```python
from build123d import *

# Parameters (mm, degrees)
SKETCH1_R           = 25
BOSS_EXTRUDE1_DEPTH = 60
CUT_EXTRUDE1_DEPTH  = 60
SKETCH2_3_R         = 25
BOSS_EXTRUDE2_DEPTH = 120.5
FILLET1_R           = 12


with BuildPart() as part:
    # Sketch1 → Boss-Extrude1 (new body)
    with BuildSketch(Plane.XY):
        with BuildLine():
            Line((60, 30), (180, 30))
            Line((180, 30), (180, -30))
            Line((180, -30), (60, -30))
            ThreePointArc((60, -30), (44.188611699, -32.565835097), (30, -40))
            ThreePointArc((30, -40), (-50, 0), (30, 40))
            ThreePointArc((30, 40), (44.188611699, 32.565835097), (60, 30))
        make_face()
        Circle(SKETCH1_R, mode=Mode.SUBTRACT)
    extrude(amount=BOSS_EXTRUDE1_DEPTH)

    # Sketch2 → Cut-Extrude1 (cut)
    with BuildSketch(Plane(origin=(180, 0, 0), x_dir=(0, 0, -1), z_dir=(1, 0, 0))):
        Polygon((-60, 11.94), (-41.94, 30), (-60, 30), align=None)
        Polygon((0, -30), (0, -11.94), (-18.06, -30), align=None)
        Polygon((0, 30), (-18.06, 30), (0, 11.94), align=None)
        Polygon((-41.94, -30), (-60, -11.94), (-60, -30), align=None)
    extrude(amount=-CUT_EXTRUDE1_DEPTH, mode=Mode.SUBTRACT)

    # Sketch2_3 → Boss-Extrude2 (add)
    with BuildSketch(Plane(origin=(180, 0, 0), x_dir=(0, 0, -1), z_dir=(1, 0, 0))):
        with Locations((-30, 0)):
            Circle(SKETCH2_3_R)
    extrude(amount=BOSS_EXTRUDE2_DEPTH)

    # Fillet1
    fillet1_edges = [part.edges().sort_by_distance(p)[0] for p in [
        (120, -20.97, 50.97),
        (120, 20.97, 9.03),
        (120, -20.97, 9.03),
        (120, 20.97, 50.97),
    ]]
    fillet(fillet1_edges, radius=FILLET1_R)


solid = part.part
```
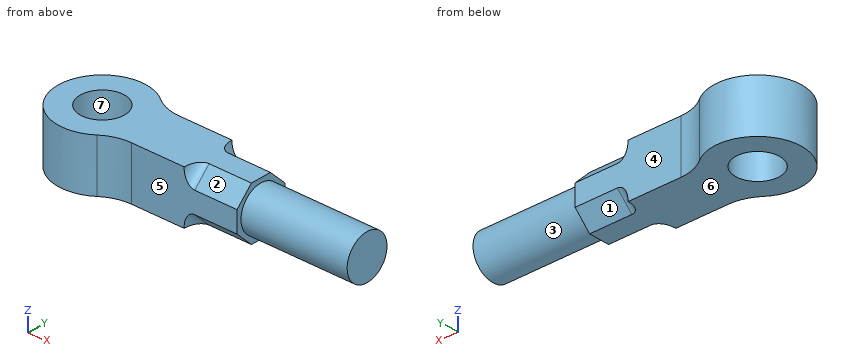
Check sheet for the modelled part. Datum: model origin and axes. Units: mm. Face numbers are marked on the shaded views. A direction names the side the tool comes from. Round coordinates to 2 decimals unless told otherwise and drop trailing zeros. Loops run counter-clockwise (first coordinate to the right, second up) from the corner with the lowest first, then second, coordinate; pieces in that order, holes last. Notation, with made-up numbers: M 79,-32.75 L 116,-32.75 A23 ccw 116,-4.75 Z; hole C 64.5,51 d6. An arc over 180 degrees is marked long. Answer as a JSON object with one key per item and string values.
1. Gauge pin test, flat ends, axial feed: P1, Ø6, axis at x = -4, y = 32, coming from the -Z side; P2, Ø3, axis at x = 188.5, y = -9, coming from the +Z side; P3, Ø5, axis at y = -8.5, z = 14.5, coming from the -X side; P4, Ø3, axis at x = 8.5, z = 47.5, coming from the -Y side. Record the tip position at first contact, or that the pin passes through.
Reply:
{"P1": "stops at z = 0", "P2": "stops at z = 53.85", "P3": "stops at x = -49.64", "P4": "stops at y = -49.51"}
2. Scan lines: line 1 (Y direction, x = 0, z = 45.5); line 2 (X direction, y = 1, z = 52); line 3 (X direction, y = -17.5, z = 28). Record each from-to range of solid material in increasing order.
Reply:
{"line 1": "y = -50 to -25, 25 to 50", "line 2": "x = -49.99 to -24.98, 24.98 to 300.5", "line 3": "x = -46.84 to -17.85, 17.85 to 300.5"}
3. Section check C-C (y = 0). Record the boundary of the cut face in (x, z), plus the area to 3 significant figures.
Reply:
{"outline": "M -50,0 L -25,0 L -25,60 L -50,60 Z; M 25,0 L 180,0 L 180,5 L 300.5,5 L 300.5,55 L 180,55 L 180,60 L 25,60 Z", "area": "16,800 mm²"}
4. Mould release check, pull along Y, two halves, no side actions. Record for the marked faces 4, 5, 6 and 7: pulls with the +Y half, pulls with the -Y half, needs draft (parallel to the pull), parting line crosses it, or undercut.
Reply:
{"face 4": "pulls with the +Y half", "face 5": "pulls with the -Y half", "face 6": "needs draft", "face 7": "undercut"}
5. Section check A-A (z = 30). Record the boundary of the cut face in (x, y), plus the area to 3 significant figures.
Reply:
{"outline": "M 30,-40 A50 cw 60,-30 L 180,-30 L 180,-25 L 300.5,-25 L 300.5,25 L 180,25 L 180,30 L 60,30 A50 cw 30,40 A50 ccw long Z; hole C 0,0 d50", "area": "20,000 mm²"}
6. Section check D-D (x = 114.5). Record the boundary of the cut face in (y, z).
Reply:
{"outline": "M -30,0 L 30,0 L 30,60 L -30,60 Z"}
7. Section check B-B (x = 0). Record the boundary of the cut face in (y, z).
Reply:
{"outline": "M -50,0 L -25,0 L -25,60 L -50,60 Z; M 25,0 L 50,0 L 50,60 L 25,60 Z"}
8. Access from +Z, -Z, +X, -X, +Y, -Y to the whole of each face (thin tool, end or side, straight path). Record for the marked faces 1, 2 and 3.
Reply:
{"face 1": "-Z, +X, +Y", "face 2": "+Z, +X, -Y", "face 3": "+X"}
